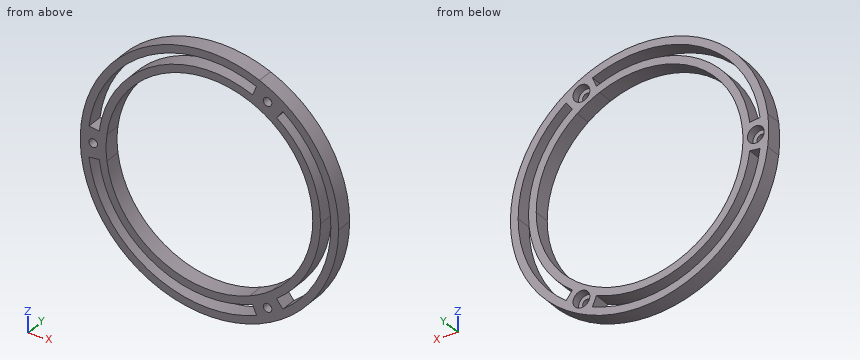
```python
from build123d import *

# Parameters (mm, degrees)
BOSS_EXTRUDE1_DEPTH = 6.35
M3_HOLES_REACH      = 72.995
SKETCH2_R           = 1.65
SKETCH3_R           = 3.25
CUT_EXTRUDE1_DEPTH  = 3.2


with BuildPart() as part:
    # Sketch1 → Boss-Extrude1 (new body)
    with BuildSketch(Plane(origin=(0, 0, 0), x_dir=(1, 0, 0), z_dir=(0, 1, 0))):
        with BuildLine():
            ThreePointArc((50, 0), (44.781853835, 22.239279825), (30.216577315, 39.83664714))
            Line((30.216577315, 39.83664714), (28.403582676, 37.446448312))
            ThreePointArc((28.403582676, 37.446448312), (42.094942605, 20.904923035), (47, 0))
            ThreePointArc((47, 0), (42.094942605, -20.904923035), (28.403582676, -37.446448312))
            Line((28.403582676, -37.446448312), (30.216577315, -39.83664714))
            ThreePointArc((30.216577315, -39.83664714), (44.781853835, -22.239279825), (50, 0))
        make_face()
        with BuildLine():
            ThreePointArc((43, 0), (38.512394298, 19.125780649), (25.986256491, 34.259516541))
            Line((25.986256491, 34.259516541), (24.173261852, 31.869317712))
            ThreePointArc((24.173261852, 31.869317712), (35.825483068, 17.79142386), (40, 0))
            ThreePointArc((40, 0), (35.825483068, -17.79142386), (24.173261852, -31.869317712))
            Line((24.173261852, -31.869317712), (25.986256491, -34.259516541))
            ThreePointArc((25.986256491, -34.259516541), (38.512394298, -19.125780649), (43, 0))
        make_face()
        with BuildLine():
            ThreePointArc((16.6764834, -39.634516541), (21.5, -37.239092363), (25.986256491, -34.259516541))
            Line((25.986256491, -34.259516541), (24.173261852, -31.869317712))
            ThreePointArc((24.173261852, -31.869317712), (20, -34.641016151), (15.513007814, -36.869317712))
            Line((15.513007814, -36.869317712), (16.6764834, -39.634516541))
        make_face()
        with BuildLine():
            ThreePointArc((18.227784182, -43.321448312), (23.5, -40.703193978), (28.403582676, -37.446448312))
            Line((28.403582676, -37.446448312), (25.986256491, -34.259516541))
            ThreePointArc((25.986256491, -34.259516541), (21.5, -37.239092363), (16.6764834, -39.634516541))
            Line((16.6764834, -39.634516541), (18.227784182, -43.321448312))
        make_face()
        with BuildLine():
            ThreePointArc((19.391259768, -46.08664714), (25, -43.301270189), (30.216577315, -39.83664714))
            Line((30.216577315, -39.83664714), (28.403582676, -37.446448312))
            ThreePointArc((28.403582676, -37.446448312), (23.5, -40.703193978), (18.227784182, -43.321448312))
            Line((18.227784182, -43.321448312), (19.391259768, -46.08664714))
        make_face()
        with BuildLine():
            ThreePointArc((-49.607837082, -6.25), (-25, -43.301270189), (19.391259768, -46.08664714))
            Line((19.391259768, -46.08664714), (18.227784182, -43.321448312))
            ThreePointArc((18.227784182, -43.321448312), (-23.5, -40.703193978), (-46.631366858, -5.875))
            Line((-46.631366858, -5.875), (-49.607837082, -6.25))
        make_face()
        with BuildLine():
            ThreePointArc((-42.662739891, -5.375), (-21.5, -37.239092363), (16.6764834, -39.634516541))
            Line((16.6764834, -39.634516541), (15.513007814, -36.869317712))
            ThreePointArc((15.513007814, -36.869317712), (-20, -34.641016151), (-39.686269666, -5))
            Line((-39.686269666, -5), (-42.662739891, -5.375))
        make_face()
        with BuildLine():
            Line((-39.686269666, 5), (-42.662739891, 5.375))
            ThreePointArc((-42.662739891, 5.375), (-43, 0), (-42.662739891, -5.375))
            Line((-42.662739891, -5.375), (-39.686269666, -5))
            ThreePointArc((-39.686269666, -5), (-40, 0), (-39.686269666, 5))
        make_face()
        with BuildLine():
            Line((-42.662739891, 5.375), (-46.631366858, 5.875))
            ThreePointArc((-46.631366858, 5.875), (-47, 0), (-46.631366858, -5.875))
            Line((-46.631366858, -5.875), (-42.662739891, -5.375))
            ThreePointArc((-42.662739891, -5.375), (-43, 0), (-42.662739891, 5.375))
        make_face()
        with BuildLine():
            Line((-46.631366858, 5.875), (-49.607837082, 6.25))
            ThreePointArc((-49.607837082, 6.25), (-50, 0), (-49.607837082, -6.25))
            Line((-49.607837082, -6.25), (-46.631366858, -5.875))
            ThreePointArc((-46.631366858, -5.875), (-47, 0), (-46.631366858, 5.875))
        make_face()
        with BuildLine():
            Line((18.227784182, 43.321448312), (19.391259768, 46.08664714))
            ThreePointArc((19.391259768, 46.08664714), (-25, 43.301270189), (-49.607837082, 6.25))
            Line((-49.607837082, 6.25), (-46.631366858, 5.875))
            ThreePointArc((-46.631366858, 5.875), (-23.5, 40.703193978), (18.227784182, 43.321448312))
        make_face()
        with BuildLine():
            Line((15.513007814, 36.869317712), (16.6764834, 39.634516541))
            ThreePointArc((16.6764834, 39.634516541), (-21.5, 37.239092363), (-42.662739891, 5.375))
            Line((-42.662739891, 5.375), (-39.686269666, 5))
            ThreePointArc((-39.686269666, 5), (-20, 34.641016151), (15.513007814, 36.869317712))
        make_face()
        with BuildLine():
            Line((24.173261852, 31.869317712), (25.986256491, 34.259516541))
            ThreePointArc((25.986256491, 34.259516541), (21.5, 37.239092363), (16.6764834, 39.634516541))
            Line((16.6764834, 39.634516541), (15.513007814, 36.869317712))
            ThreePointArc((15.513007814, 36.869317712), (20, 34.641016151), (24.173261852, 31.869317712))
        make_face()
        with BuildLine():
            Line((25.986256491, 34.259516541), (28.403582676, 37.446448312))
            ThreePointArc((28.403582676, 37.446448312), (23.5, 40.703193978), (18.227784182, 43.321448312))
            Line((18.227784182, 43.321448312), (16.6764834, 39.634516541))
            ThreePointArc((16.6764834, 39.634516541), (21.5, 37.239092363), (25.986256491, 34.259516541))
        make_face()
        with BuildLine():
            Line((28.403582676, 37.446448312), (30.216577315, 39.83664714))
            ThreePointArc((30.216577315, 39.83664714), (25, 43.301270189), (19.391259768, 46.08664714))
            Line((19.391259768, 46.08664714), (18.227784182, 43.321448312))
            ThreePointArc((18.227784182, 43.321448312), (23.5, 40.703193978), (28.403582676, 37.446448312))
        make_face()
    extrude(amount=BOSS_EXTRUDE1_DEPTH)

    # Sketch2 → M3-holes (cut, up to next)
    with BuildSketch(Plane(origin=(0, 6.35, 0), x_dir=(1, 0, 0), z_dir=(0, 1, 0)), mode=Mode.PRIVATE) as m3_holes_sk1:
        with Locations(Location((-45, 0, 0), (0, 0, 270))):
            Circle(SKETCH2_R)
    m3_holes_tool1 = extrude(m3_holes_sk1.sketch, amount=-M3_HOLES_REACH, mode=Mode.PRIVATE) & part.part
    # Sketch2 → M3-holes (cut, up to next)
    with BuildSketch(Plane(origin=(0, 6.35, 0), x_dir=(1, 0, 0), z_dir=(0, 1, 0)), mode=Mode.PRIVATE) as m3_holes_sk2:
        with Locations(Location((22.5, -38.97114317, 0), (0, 0, 270))):
            Circle(SKETCH2_R)
    m3_holes_tool2 = extrude(m3_holes_sk2.sketch, amount=-M3_HOLES_REACH, mode=Mode.PRIVATE) & part.part
    # Sketch2 → M3-holes (cut, up to next)
    with BuildSketch(Plane(origin=(0, 6.35, 0), x_dir=(1, 0, 0), z_dir=(0, 1, 0)), mode=Mode.PRIVATE) as m3_holes_sk3:
        with Locations(Location((22.5, 38.97114317, 0), (0, 0, 270))):
            Circle(SKETCH2_R)
    m3_holes_tool3 = extrude(m3_holes_sk3.sketch, amount=-M3_HOLES_REACH, mode=Mode.PRIVATE) & part.part
    add(m3_holes_tool1.solids().sort_by_distance((-45, 6.35, 0))[0], mode=Mode.SUBTRACT)
    add(m3_holes_tool2.solids().sort_by_distance((22.5, 6.35, 38.971143))[0], mode=Mode.SUBTRACT)
    add(m3_holes_tool3.solids().sort_by_distance((22.5, 6.35, -38.971143))[0], mode=Mode.SUBTRACT)

    # Sketch3 → Cut-Extrude1 (cut)
    with BuildSketch(Plane(origin=(0, 6.35, 0), x_dir=(1, 0, 0), z_dir=(0, 1, 0))):
        with Locations(Location((-45, 0, 0), (0, 0, 270))):
            Circle(SKETCH3_R)
        with Locations(Location((22.5, 38.97114317, 0), (0, 0, 270))):
            Circle(SKETCH3_R)
        with Locations(Location((22.5, -38.97114317, 0), (0, 0, 270))):
            Circle(SKETCH3_R)
    extrude(amount=-CUT_EXTRUDE1_DEPTH, mode=Mode.SUBTRACT)


solid = part.part
```
Design review of the part built by this model. Coordinates are the model's own, in mm. Round coordinates to 2 decimals unless told otherwise and drop trailing zeros. Order: outer loops, then holes, each group sorted by start corner. A loop starts at its lowest first (then second) coordinate and runs counter-clockwise, first axis right, second up. Notation, with made-up numbers: (43, 47) - (53, 47) arc R28 cw to (53, 68) - close; hole circle Ø3 at (56.25, 57). An arc over 180 degrees is marked (long way). One line per question, with ' | ' between items.
Item 1: Take a section at C-C, the plane z = -18. Write out the cut boundary in (x, y).
Checks:
outline: (-46.65, 0) - (-43.42, 0) - (-43.42, 6.35) - (-46.65, 6.35) - close; (-39.05, 0) - (-35.72, 0) - (-35.72, 6.35) - (-39.05, 6.35) - close; (35.72, 0) - (39.05, 0) - (39.05, 6.35) - (35.72, 6.35) - close; (43.42, 0) - (46.65, 0) - (46.65, 6.35) - (43.42, 6.35) - close
Item 2: Take a section at B-B, the plane x = 22.5. Write out the cut boundary in (y, z).
Checks:
outline: (0, -44.65) - (6.35, -44.65) - (6.35, -42.22) - (3.15, -42.22) - (3.15, -40.62) - (0, -40.62) - close; (0, -37.32) - (3.15, -37.32) - (3.15, -35.72) - (6.35, -35.72) - (6.35, -33.07) - (0, -33.07) - close; (0, 33.07) - (6.35, 33.07) - (6.35, 35.72) - (3.15, 35.72) - (3.15, 37.32) - (0, 37.32) - close; (0, 40.62) - (3.15, 40.62) - (3.15, 42.22) - (6.35, 42.22) - (6.35, 44.65) - (0, 44.65) - close
Item 3: Take a section at A-A, the plane y = 5. Write out the cut boundary in (x, z) (3 decimals).
Checks:
outline: circle Ø100 at (0, 0); hole circle Ø6.5 at (-45, 0); hole (-46.631, -5.875) arc R47 ccw to (18.228, -43.321) - (16.676, -39.635) arc R43 cw to (-42.663, -5.375) - close; hole (-46.631, 5.875) - (-42.663, 5.375) arc R43 cw to (16.676, 39.635) - (18.228, 43.321) arc R47 ccw to start; hole circle Ø80 at (0, 0); hole circle Ø6.5 at (22.5, -38.971); hole circle Ø6.5 at (22.5, 38.971); hole (25.986, -34.26) - (28.404, -37.446) arc R47 ccw to (28.404, 37.446) - (25.986, 34.26) arc R43 cw to start
Item 4: Take a section at D-D, the plane x = -23. Write out the cut boundary in (y, z), then the cut area to 3 significant figures.
Checks:
outline: (0, -44.4) - (6.35, -44.4) - (6.35, -40.99) - (0, -40.99) - close; (0, -36.33) - (6.35, -36.33) - (6.35, -32.73) - (0, -32.73) - close; (0, 32.73) - (6.35, 32.73) - (6.35, 36.33) - (0, 36.33) - close; (0, 40.99) - (6.35, 40.99) - (6.35, 44.4) - (0, 44.4) - close | area: 89.1 mm²
Item 5: Wall thickness on line 1 (X direction, y = 5.75, z = -9.5); line 2 (X direction, y = 1.75, z = -12.5); line 3 (X direction, y = 0.5, z = -2): over which ranges is each line inside the solid? List them lowest first. Write a range as [from, to].
Checks:
line 1: [-49.09, -46.03], [-41.94, -38.86], [38.86, 41.94], [46.03, 49.09] | line 2: [-48.41, -45.31], [-41.14, -38], [38, 41.14], [45.31, 48.41] | line 3: [-49.96, -39.95], [39.95, 42.95], [46.96, 49.96]
Item 6: For P1, Ø4.5, axis at x = 22.5, z = -38.97, coming from the +Y side; P2, Ø2, axis at x = 22.5, z = 38.97, coming from the +Y side; P3, Ø10.5, axis at x = 22.5, z = 38.97, coming from the -Y side; P4, Ø2, axis at x = -32, y = 0.5, coming from the +Z side, all flat-tipped, find the tip position at first contact; note any pin that passes through.
Checks:
P1: y = 3.15 | P2: through | P3: y = 0 | P4: z = 39.23
